```python
from build123d import *

# Parameters (mm, degrees)
SKETCH_1_W          = 45
SKETCH_1_H          = 50
SKETCH_1_R          = 1.6
SKETCH_1_R_2        = 2.1
EXTRUDE_1_DEPTH     = 4
FILLET_1_R          = 2
FILLET_2_R          = 10
CUT_EXTRUDE_1_DEPTH = 10
FILLET_3_R          = 2
SKETCH_3_W          = 5.729916775
SKETCH_3_H          = 6
CUT_EXTRUDE_2_DEPTH = 10
CUT_EXTRUDE_3_DEPTH = 10
FILLET_4_R          = 2
CUT_EXTRUDE_4_DEPTH = 10
FILLET_5_R          = 2
CUT_EXTRUDE_5_DEPTH = 10
SKETCH_8_R          = 1.6
CUT_EXTRUDE_6_DEPTH = 10
SKETCH_9_R          = 1.6
CUT_EXTRUDE_7_DEPTH = 10
FILLET_8_R          = 2


with BuildPart() as part:
    # 草图1 → 凸台-拉伸1 (new body)
    # profile 1 of 3: a face of its own
    with BuildSketch(Plane.XY):
        Polygon((-102.5, 25), (-102.5, 19), (-22.5, 0), (-22.5, 25), align=None)
    # profile 2 of 3: a face of its own
    with BuildSketch(Plane.XY):
        Rectangle(SKETCH_1_W, SKETCH_1_H)
        with Locations((-6, -6)):
            Circle(SKETCH_1_R, mode=Mode.SUBTRACT)
        with Locations((6, -6)):
            Circle(SKETCH_1_R, mode=Mode.SUBTRACT)
        with Locations((6, 6)):
            Circle(SKETCH_1_R, mode=Mode.SUBTRACT)
        with Locations((-6, 6)):
            Circle(SKETCH_1_R, mode=Mode.SUBTRACT)
        with Locations((-16.5, -20)):
            Circle(SKETCH_1_R_2, mode=Mode.SUBTRACT)
        with Locations((16.5, -20)):
            Circle(SKETCH_1_R_2, mode=Mode.SUBTRACT)
        with Locations((16.5, 20)):
            Circle(SKETCH_1_R_2, mode=Mode.SUBTRACT)
        with Locations((-16.5, 20)):
            Circle(SKETCH_1_R_2, mode=Mode.SUBTRACT)
    # profile 3 of 3: a face of its own
    with BuildSketch(Plane.XY):
        Polygon((92.5, 25), (22.5, 25), (22.5, 0), (92.5, 19), align=None)
    extrude(amount=EXTRUDE_1_DEPTH)

    # 圆角1
    fillet_1_edges = [part.edges().sort_by_distance(p)[0] for p in [
        (92.5, 25, 2),
        (92.5, 19, 2),
        (22.5, -25, 2),
        (-22.5, -25, 2),
        (-102.5, 19, 2),
        (-102.5, 25, 2),
    ]]
    fillet(fillet_1_edges, radius=FILLET_1_R)

    # 圆角2
    fillet_2_edges = [part.edges().sort_by_distance(p)[0] for p in [
        (22.5, 0, 2),
        (-22.5, 0, 2),
    ]]
    fillet(fillet_2_edges, radius=FILLET_2_R)

    # 草图2 → 切除-拉伸1 (cut)
    with BuildSketch(Plane.XY.offset(4)):
        Polygon((-10, 19), (10, 19), (0, 7), align=None)
        Polygon((0, -7), (-10, -19), (10, -19), align=None)
    extrude(amount=-CUT_EXTRUDE_1_DEPTH, mode=Mode.SUBTRACT)

    # 圆角3
    fillet_3_edges = [part.edges().sort_by_distance(p)[0] for p in [
        (0, 7, 2),
        (-10, 19, 2),
        (10, 19, 2),
        (10, -19, 2),
        (-10, -19, 2),
        (0, -7, 2),
    ]]
    fillet(fillet_3_edges, radius=FILLET_3_R)

    # 草图3 → 切除-拉伸2 (cut)
    with BuildSketch(Plane(origin=(0, 0, 0), x_dir=(-1, 0, 0), z_dir=(0, 0, -1))):
        with Locations((2.864958388, 22)):
            Rectangle(SKETCH_3_W, SKETCH_3_H)
        with Locations((-2.864958388, 22)):
            Rectangle(SKETCH_3_W, SKETCH_3_H)
        with Locations((2.864958388, -22)):
            Rectangle(SKETCH_3_W, SKETCH_3_H)
        with Locations((-2.864958388, -22)):
            Rectangle(SKETCH_3_W, SKETCH_3_H)
    extrude(amount=-CUT_EXTRUDE_2_DEPTH, mode=Mode.SUBTRACT)

    # 草图4 → 切除-拉伸3 (cut)
    with BuildSketch(Plane(origin=(0, 0, 0), x_dir=(-1, 0, 0), z_dir=(0, 0, -1))):
        with BuildLine():
            Line((-5.729916775, 25), (-7.729916775, 25))
            Line((-7.729916775, 25), (-7.729916775, 17))
            ThreePointArc((-7.729916775, 17), (-7.144130337, 18.414213562), (-5.729916775, 19))
            Line((-5.729916775, 19), (-5.729916775, 25))
        make_face()
        with BuildLine():
            Line((7.729916775, 25), (5.729916775, 25))
            Line((5.729916775, 25), (5.729916775, 19))
            ThreePointArc((5.729916775, 19), (7.144130337, 18.414213562), (7.729916775, 17))
            Line((7.729916775, 17), (7.729916775, 25))
        make_face()
        with BuildLine():
            Line((-7.729916775, -17), (-7.729916775, -25))
            Line((-7.729916775, -25), (-5.729916775, -25))
            Line((-5.729916775, -25), (-5.729916775, -19))
            ThreePointArc((-5.729916775, -19), (-7.144130337, -18.414213562), (-7.729916775, -17))
        make_face()
        with BuildLine():
            Line((5.729916775, -19), (5.729916775, -25))
            Line((5.729916775, -25), (7.729916775, -25))
            Line((7.729916775, -25), (7.729916775, -17))
            ThreePointArc((7.729916775, -17), (7.144130337, -18.414213562), (5.729916775, -19))
        make_face()
    extrude(amount=-CUT_EXTRUDE_3_DEPTH, mode=Mode.SUBTRACT)

    # 圆角4
    fillet_4_edges = [part.edges().sort_by_distance(p)[0] for p in [
        (7.729916775, 25, 2),
        (-7.729916775, 25, 2),
        (-7.729916775, -25, 2),
        (7.729916775, -25, 2),
    ]]
    fillet(fillet_4_edges, radius=FILLET_4_R)

    # 草图6 → 切除-拉伸4 (cut)
    with BuildSketch(Plane.XY.offset(4)):
        Polygon((6.5, 0), (16.5, 10), (16.5, -10), align=None)
        Polygon((-6.5, 0), (-16.5, -10), (-16.5, 10), align=None)
    extrude(amount=-CUT_EXTRUDE_4_DEPTH, mode=Mode.SUBTRACT)

    # 圆角5
    fillet_5_edges = [part.edges().sort_by_distance(p)[0] for p in [
        (16.5, -10, 2),
        (6.5, 0, 2),
        (16.5, 10, 2),
        (-16.5, 10, 2),
        (-6.5, 0, 2),
        (-16.5, -10, 2),
    ]]
    fillet(fillet_5_edges, radius=FILLET_5_R)

    # 草图7 → 切除-拉伸5 (cut)
    with BuildSketch(Plane.XY.offset(4)):
        Polygon((-85.07228941, 20), (-24.5, 5.614081265), (-24.5, 20), align=None)
        Polygon((24.5, 20), (24.5, 5.723767945), (77.096644415, 20), align=None)
    extrude(amount=-CUT_EXTRUDE_5_DEPTH, mode=Mode.SUBTRACT)

    # 草图8 → 切除-拉伸6 (cut)
    with BuildSketch(Plane.XY.offset(4)):
        with Locations((-97.5, 22)):
            Circle(SKETCH_8_R)
        with Locations((-77.5, 22)):
            Circle(SKETCH_8_R)
    extrude(amount=-CUT_EXTRUDE_6_DEPTH, mode=Mode.SUBTRACT)

    # 草图9 → 切除-拉伸7 (cut)
    with BuildSketch(Plane.XY.offset(4)):
        with Locations((87.5, 22)):
            Circle(SKETCH_9_R)
        with Locations((67.5, 22)):
            Circle(SKETCH_9_R)
    extrude(amount=-CUT_EXTRUDE_7_DEPTH, mode=Mode.SUBTRACT)

    # 圆角8
    fillet_8_edges = [part.edges().sort_by_distance(p)[0] for p in [
        (-85.07228941, 20, 2),
        (-24.5, 20, 2),
        (-24.5, 5.614081265, 2),
        (24.5, 20, 2),
        (77.096644415, 20, 2),
        (24.5, 5.723767945, 2),
    ]]
    fillet(fillet_8_edges, radius=FILLET_8_R)


solid = part.part
```
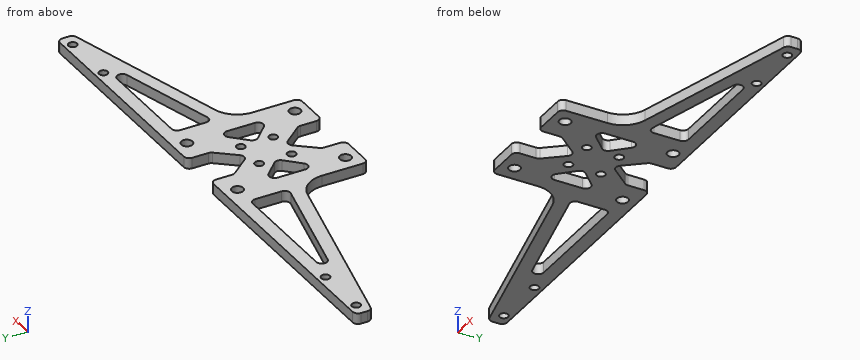
Input: part model. Units: mm. Frame: model coordinates. Give positions to 0.01 mm unless a question says otherwise; leave off trailing zeros. Order: outer loops, then holes, each group sorted by start corner. A loop starts at its lowest first (then second) coordinate and runs counter-clockwise, first axis right, second up. Notation, with made-up numbers: M -17,87 L 13,87 A25 cw 13,120 Z; hole C -36.75,-29.75 d11. An arc over 180 degrees is marked long. Return JSON: item names as keys, results as strings.
Item 1: First-contact query: P1, Ø2, axis at y = -16, z = 2, coming from the -X side; P2, Ø1.2, axis at x = -51.5, z = 1, coming from the -Y side (3 decimals); P3, Ø2, axis at y = -17, z = 2.5, coming from the +X side. Flat tips, straight axial feed; report the tip coordinate or a pass-through.
Solutions:
{"P1": "x = -22.5", "P2": "y = 6.745", "P3": "x = 22.5"}
Item 2: Cut plane A-A (y = -13). Return loops of the section in (x, z), then the cut area to 3 significant figures.
Solutions:
{"outline": "M -22.5,0 L -5,0 L -5,4 L -22.5,4 Z; M 5,0 L 22.5,0 L 22.5,4 L 5,4 Z", "area": "140 mm^2"}
Item 3: Cut plane B-B (x = 55). Return loops of the section in (y, z).
Solutions:
{"outline": "M 8.82,0 L 14,0 L 14,4 L 8.82,4 Z; M 20,0 L 25,0 L 25,4 L 20,4 Z"}
Item 4: Cut plane D-D (x = -90). Return loops of the section in (y, z).
Solutions:
{"outline": "M 16.03,0 L 25,0 L 25,4 L 16.03,4 Z"}
Item 5: Cut plane C-C (z = 3.25). State how many separate pieces and enclosed holes the cut face has, then the cut area to 3 significant figures.
Solutions:
{"separate pieces": "1", "enclosed holes": "16", "area": "3,130 mm^2"}
Item 6: Ray query, probe 1 along X at (y, z) = (-21.5, 1.5); probe 2 along Y at (x, z) = (-18, 2.6); probe 3 along X at (y, z) = (-7, 3.7). Return the intervals inside material, ascending.
Solutions:
{"probe 1": "-22.5 to -17.97, -15.03 to -7.73, 7.73 to 15.03, 17.97 to 22.5", "probe 2": "-25 to -21.47, -18.53 to 18.53, 21.47 to 25", "probe 3": "-22.54 to -15.31, -13.69 to -7.25, -4.75 to 4.75, 7.25 to 13.69, 15.31 to 22.52"}
